Input: part model. Units: mm. Frame: model coordinates. A direction names the side the tool comes from. Give positions to 0.01 mm unless a question says otherwise; leave off trailing zeros. Order: outer loops, then holes, each group sorted by start corner. A loop starts at its lowest first (then second) coordinate and runs counter-clockwise, first axis right, second up. Notation, with made-up numbers: (38.25, 43.5) - (97.25, 43.5) arc R28 ccw to (97.25, 70.5) - close; hole circle Ø5 at (-21.5, 56). An arc over 180 degrees is marked (long way). Use a Markdown table: item, result.
from build123d import *

# Parameters (mm, degrees)
SKETCH1_W           = 13.97
SKETCH1_H           = 12.7
BOSS_EXTRUDE1_DEPTH = 2.54
FILLET1_R           = 0.635
SHELL1_START        = 0.635
SHELL1_OUTLINE_W    = 1.905
SHELL1_OUTLINE_H    = 11.43
SHELL1_DEPTH        = 12.7
SKETCH2_R           = 2.54
BOSS_EXTRUDE2_DEPTH = 1.905
BOSS_EXTRUDE4_DEPTH = 0.00254


# Read off the part's stored shape, not the designer's step: Shell1
with BuildPart() as part:
    # Sketch1 → Boss-Extrude1 (new body)
    with BuildSketch(Plane(origin=(0, 0, 0), x_dir=(1, 0, 0), z_dir=(0, 1, 0))):
        with Locations((6.985, 6.35)):
            Rectangle(SKETCH1_W, SKETCH1_H)
    extrude(amount=BOSS_EXTRUDE1_DEPTH)

    # Fillet1
    fillet1_edges = [part.edges().sort_by_distance(p)[0] for p in [
        (0, 1.27, -12.7),
        (13.97, 1.27, -12.7),
        (13.97, 1.27, 0),
        (0, 1.27, 0),
    ]]
    fillet(fillet1_edges, radius=FILLET1_R)

    # Shell1 outline → Shell1 (cut)
    with BuildSketch(Plane.YZ.offset(SHELL1_START)):
        with Locations((0.9525, -6.35)):
            Rectangle(SHELL1_OUTLINE_W, SHELL1_OUTLINE_H)
    extrude(amount=SHELL1_DEPTH, mode=Mode.SUBTRACT)

    # Sketch2 → Boss-Extrude2 (add)
    with BuildSketch(Plane(origin=(0, 1.905, 0), x_dir=(-1, 0, 0), z_dir=(0, -1, 0))):
        with Locations(Location((-6.985, 6.35, 0), (0, 0, 270))):
            Circle(SKETCH2_R)
    extrude(amount=BOSS_EXTRUDE2_DEPTH)

    # Sketch5 → Boss-Extrude4 (add)
    with BuildSketch(Plane(origin=(0, 2.54, 0), x_dir=(1, 0, 0), z_dir=(0, 1, 0))):
        Polygon((3.675799971, 8.636881907), (6.405771964, 8.963367107), (6.405771964, 6.385040601), (3.675799971, 6.385040601), align=None)
        Polygon((3.675799971, 6.099704546), (3.675799971, 4.006611728), (6.405771964, 3.488506251), (6.405771964, 6.099704546), align=None)
        Polygon((6.706531591, 8.999335816), (6.706531591, 6.385040601), (10.345846979, 6.385040601), (10.345846979, 9.434572007), align=None)
        Polygon((6.706531591, 6.099704546), (6.706531591, 3.431426834), (10.345846979, 2.740742373), (10.345846979, 6.099704546), align=None)
    extrude(amount=BOSS_EXTRUDE4_DEPTH)


solid = part.part
1. Section query B-B (z = -11). Return loops of the section in (x, y) (3 decimals), then the cut area to 3 significant figures.
Response:
| item | result |
|---|---|
| outline | (0, 0) - (0.635, 0) - (0.635, 1.905) - (13.335, 1.905) - (13.335, 0) - (13.97, 0) - (13.97, 2.54) - (0, 2.54) - close |
| area | 11.3 mm^2 |
2. Section query A-A (y = 1.15). Return loops of the section in (x, z) (3 decimals), then the cut area to 3 significant figures.
Response:
| item | result |
|---|---|
| outline | (0, -12.065) arc R0.635 ccw to (0.635, -12.7) - (13.335, -12.7) arc R0.635 ccw to (13.97, -12.065) - (13.97, -0.635) arc R0.635 ccw to (13.335, 0) - (0.635, 0) arc R0.635 ccw to (0, -0.635) - close; circle Ø5.08 at (6.985, -6.35); hole (0.635, -12.065) - (13.335, -12.065) - (13.335, -0.635) - (0.635, -0.635) - close |
| area | 52.2 mm^2 |
3. Set-up query: faces 1 (the face through (13.97, 1, -6)), 2 (the face through (4, 1.905, -6)). Return all of +Z, -Z, +X, -X, +Y, -Y with unobstructed straight access to the full face (end or side cutting, diameter ignored); none if empty.
Response:
| item | result |
|---|---|
| face 1 | +Z, -Z, +X, +Y, -Y |
| face 2 | -Y |
4. Pin query (flat end, axial travel): pin 1 (1.5 mm diameter, centred on x = 2, z = -8, fed in from +Y). Return the tip coordinate at first contact, or that it passes through.
Response:
| item | result |
|---|---|
| pin 1 | stops at y = 2.54 |
5. Material intervals for line 1 along Z through (x, y) = (7, 0.7) (3 decimals); line 2 along X through (y, z) = (1.7, -1.75) (3 decimals); line 3 along Z through (x, y) = (1, 1.1) (3 decimals), sorted ascending.
Response:
| item | result |
|---|---|
| line 1 | z = -12.7 to -12.065, -8.89 to -3.81, -0.635 to 0 |
| line 2 | x = 0 to 0.635, 13.335 to 13.97 |
| line 3 | z = -12.7 to -12.065, -0.635 to 0 |
6. Section query C-C (x = 2). Return loops of the section in (y, z) (3 decimals), then the cut area to 3 significant figures.
Response:
| item | result |
|---|---|
| outline | (0, -12.7) - (2.54, -12.7) - (2.54, 0) - (0, 0) - (0, -0.635) - (1.905, -0.635) - (1.905, -12.065) - (0, -12.065) - close |
| area | 10.5 mm^2 |
7. Mould query, pull axis Z, two halves, no side actions, for faces 3 (the face through (0.635, 1, -6)), 4 (the face through (9, 2.543, -8)), 5 (the face through (7, 1, -12.7)). Classes: pulls with the +Z half, pulls with the -Z half, needs draft (parallel to the pull), parting line crosses it, or undercut.
Response:
| item | result |
|---|---|
| face 3 | undercut |
| face 4 | needs draft |
| face 5 | pulls with the -Z half |
